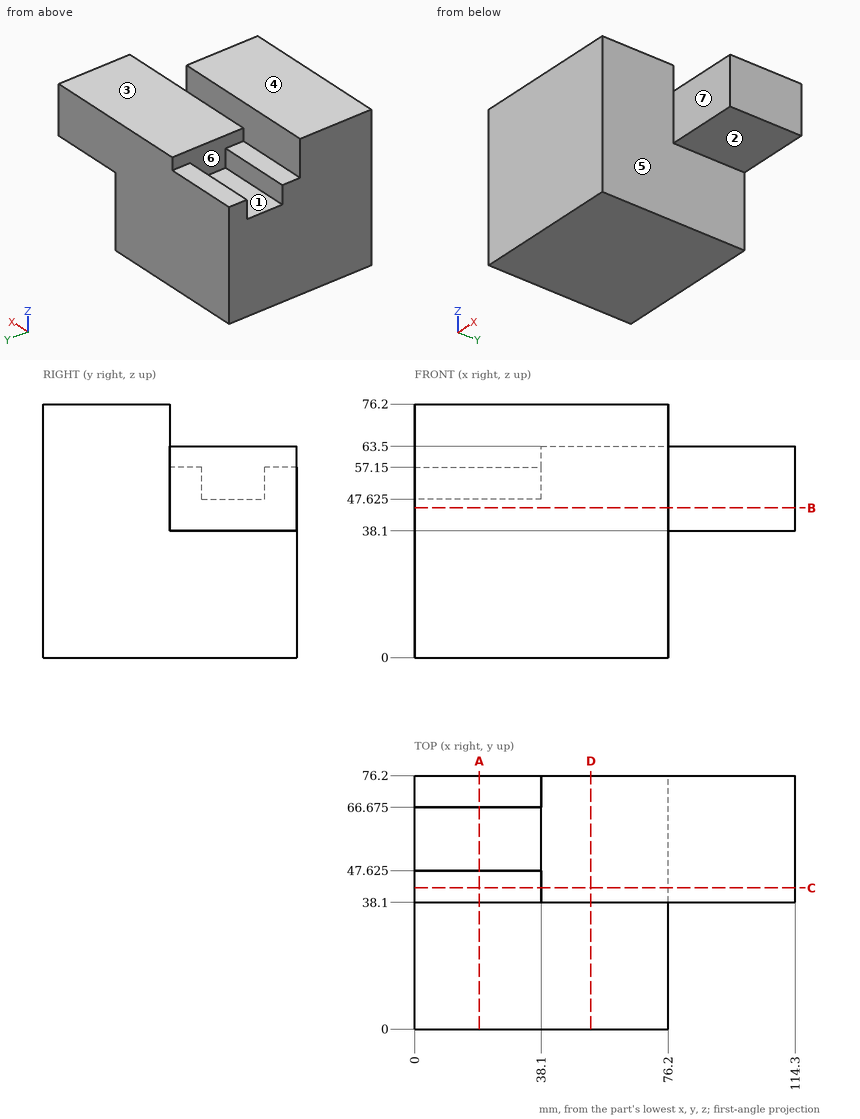
Here's the drawing with two shaded views (mm, measured from the low corner). I have some questions. A direction names the side the tool comes from. Coordinates: 2 decimals unless noted, no trailing zeros. Loops run counter-clockwise (first coordinate to the right, second up) from the corner with the lowest first, then second, coordinate; pieces in that order, holes last. Notation, with made-up numbers: M -21.75,59.5 L -8.75,59.5 A16 ccw -8.75,80.5 Z; hole C 49.25,-7 d2. An arc over 180 degrees is marked long. Put each result on its own line as item: value. Start each with the question number.
(1) Imagine slicing it at A-A on x = 19.5. List the corners of the cut face in (y, z) for me (3 decimals), and give its area (3 significant figures).
(2) Which directions (+Z, -Z, +X, -X, +Y, -Y) give clear straight access to the entire face, cutting with the end or side of a thin tool? Please do the marked faces 1, 2, 3 and 4.
(3) We'd pull the mould along Y, two halves only. Please class the marked faces 5, 6 and 7: +Y half, -Y half, draft (parallel to the pull), parting line (faces both ways), or undercut.
(4) Will these pins go through, and if not, where does the flat tip stop? pin 1 Ø15 at (x, y) = (18, 60.5) entering from +Z; pin 2 Ø8 at (y, z) = (54, 19.5) entering from +X; pin 3 Ø7.5 at (x, z) = (103, 48) entering from -Y; pin 4 Ø5 at (x, y) = (88.5, 34) entering from -Z.
(5) Imagine slicing it at C-C on y = 42.5. List the corners of the cut face in (x, z) for me.
(6) Imagine slicing it at B-B on z = 45. List the corners of the cut face in (x, y) for me, and give its area (3 significant figures).
(7) Imagine slicing it at D-D on x = 53. List the corners of the cut face in (y, z) for me, and give its area (3 significant figures).
(8) I need wall thicknesses on probe 1 along X at (y, z) = (52.5, 53.5); probe 2 along Z at (x, y) = (11, 67); probe 3 along Z at (x, y) = (105, 62.5). Which ranges of each line are inside material? Lowest first, please.
Worked answers:
1. outline: M 0,0 L 76.2,0 L 76.2,57.15 L 66.675,57.15 L 66.675,47.625 L 47.625,47.625 L 47.625,57.15 L 38.1,57.15 L 38.1,76.2 L 0,76.2 Z
1. area: 4,900 mm2
2. face 1: +Z, -X
2. face 2: -Z, +X, +Y, -Y
2. face 3: +Z, +X, -X, +Y
2. face 4: +Z, +X, -X, +Y, -Y
3. face 5: draft
3. face 6: undercut
3. face 7: -Y half
4. pin 1: stops at z = 57.15
4. pin 2: stops at x = 76.2
4. pin 3: stops at y = 38.1
4. pin 4: passes through
5. outline: M 0,0 L 76.2,0 L 76.2,38.1 L 114.3,38.1 L 114.3,63.5 L 38.1,63.5 L 38.1,57.15 L 0,57.15 Z
6. outline: M 0,0 L 76.2,0 L 76.2,38.1 L 114.3,38.1 L 114.3,76.2 L 0,76.2 Z
6. area: 7,260 mm2
7. outline: M 0,0 L 76.2,0 L 76.2,63.5 L 38.1,63.5 L 38.1,76.2 L 0,76.2 Z
7. area: 5,320 mm2
8. probe 1: x = 38.1 to 114.3
8. probe 2: z = 0 to 57.15
8. probe 3: z = 38.1 to 63.5
